from build123d import *

# Parameters (mm, degrees)
PAD_START          = -51
SKETCH_R           = 20
SKETCH_R_2         = 18.4
PAD_DEPTH          = 18
SKETCH001_R        = 21
PAD001_DEPTH       = 1
SKETCH002_R        = 4
PAD002_DEPTH       = 8.8
POCKET_DEPTH       = 9.801
PAD003_DEPTH       = 0.5
PAD003_DEPTH_BACK  = 0.5
POLARPATTERN_COUNT = 6


with BuildPart() as part:
    # Sketch → Pad (new body)
    with BuildSketch(Plane.XZ.offset(PAD_START)):
        Circle(SKETCH_R)
        Circle(SKETCH_R_2, mode=Mode.SUBTRACT)
    extrude(amount=-PAD_DEPTH)

    # Sketch001 (on Face3 of Pad) → Pad001 (join)
    with BuildSketch(Plane(origin=(0, 69, 0), x_dir=(1, 0, 0), z_dir=(0, 1, 0))):
        Circle(SKETCH001_R)
    extrude(amount=PAD001_DEPTH)

    # Sketch002 (on Face7 of Pad001) → Pad002 (join)
    with BuildSketch(Plane.XZ.offset(-69)):
        Circle(SKETCH002_R)
    extrude(amount=PAD002_DEPTH)

    # Sketch003 (on Face9 of Pad002) → Pocket (cut, through all)
    with BuildSketch(Plane.XZ.offset(-60.2)):
        with BuildLine():
            ThreePointArc((-1.249, 1), (-1.548005, -0.404574), (-0.6, -1.48324))
            Line((-0.6, -1.48324), (-0.6, -13.48324))
            Line((-0.6, -13.48324), (0.6, -13.48324))
            Line((0.6, -13.48324), (0.6, -1.48324))
            ThreePointArc((0.6, -1.48324), (1.548005, -0.404574), (1.249, 1))
            Line((-1.249, 1), (1.249, 1))
        make_face()
    extrude(amount=-POCKET_DEPTH, mode=Mode.SUBTRACT)

    # Sketch004 → Pad003 (join, two sides)
    with BuildSketch(Plane.XY) as pad003_sk:
        with BuildLine():
            ThreePointArc((-4, 60.2), (-5.757359, 64.442641), (-10, 66.2))
            ThreePointArc((-12.196813, 66.402796), (-11.103077, 66.250807), (-10, 66.2))
            Line((-19.7, 67.8), (-12.196813, 66.402796))
            Line((-19.7, 69), (-19.7, 67.8))
            Line((-19.7, 69), (-3.5, 69))
            Line((-3.5, 69), (-3.5, 60.2))
            Line((-3.5, 60.2), (-4, 60.2))
        make_face()
    pad003 = extrude(amount=PAD003_DEPTH) + extrude(pad003_sk.sketch, amount=-PAD003_DEPTH_BACK)

    # PolarPattern: Pad003 ×6 about axis
    polarpattern_axis = Axis((0, 0, 0), (0, 1, 0))
    for i in range(1, POLARPATTERN_COUNT):
        add(pad003.rotate(polarpattern_axis, i * 360 / POLARPATTERN_COUNT))


solid = part.part
The model under review builds one solid part; all positions refer to its coordinate system, in mm. A direction names the side the tool comes from. Give positions to 0.01 mm unless a question says otherwise; leave off trailing zeros. Write each loop counter-clockwise with the first axis right and the second up, starting at its lowest first coordinate (ties: lowest second). Pieces come first, ordered by that corner, then holes.
1. Add section A-A, the plane z = 0. Write out the cut boundary in (x, y).
2. Add section C-C, the plane y = 60.75. Count the separate pieces of the cut face and the enclosed holes in it, plus the area to 3 significant figures.
3. Wall thickness on L1, parallel to Z at x = 0, y = 60.5; L2, parallel to Z at x = 1, y = 66.5; L3, parallel to Z at x = 0, y = 58.5: over which ranges is each line inside the solid? List them lowest first.
4. Add section B-B, the plane x = 0. Write out the cut boundary in (y, z), plus the area to 3 significant figures.
5. Tool access review of faces 1 (the flat face through (-0.2, 60.2, 1.2)), 2 (the flat face through (18, 51, -6)), 3 (the flat face through (0, 69.5, -13.483)): name each direction out of +Z, -Z, +X, -X, +Y, -Y from which nothing blocks a thin tool from reaching the whole face with its end or side.
6. For P1, Ø5, axis at x = 7.5, y = 57.5, coming from the -Z side; P2, Ø2.5, axis at x = 13.5, y = 64, coming from the -Z side; P3, Ø4.5, axis at x = 3, z = 9.5, coming from the -Y side, all flat-tipped, find the tip position at first contact; note any pin that passes through.
7. Draft analysis for pull direction X (two halves, no side actions). For faces 4 (the cylindrical face through (-4.336, 59.874, -19.524)), 5 (the flat face through (-5.21, 67.23, 8.02)), 6 (the flat face through (0, 70, 4)), state which applies: +X half, -X half, draft (parallel to the pull), parting line (faces both ways), or undercut.
Worked answers:
1. outline: (-21, 69) - (-20, 69) - (-20, 51) - (-18.4, 51) - (-18.4, 67.56) - (-12.2, 66.4) arc R12 ccw to (-10, 66.2) arc R6 cw to (-4, 60.2) - (-1.6, 60.2) - (-1.6, 70) - (-21, 70) - close; (1.6, 60.2) - (4, 60.2) arc R6 cw to (10, 66.2) arc R12 ccw to (12.2, 66.4) - (18.4, 67.56) - (18.4, 51) - (20, 51) - (20, 69) - (21, 69) - (21, 70) - (1.6, 70) - close
2. separate pieces: 2
2. enclosed holes: 1
2. area: 234 mm2
3. L1: z = -20 to -18.4, 1 to 4, 18.4 to 20
3. L2: z = -19.97 to -18.37, -3.87 to -1.25, 1 to 3.87, 18.37 to 19.97
3. L3: z = -20 to -18.4, 18.4 to 20
4. outline: (51, -20) - (69, -20) - (69, -21) - (70, -21) - (70, -13.48) - (69, -13.48) - (69, -18.4) - (51, -18.4) - close; (51, 18.4) - (69, 18.4) - (69, 4) - (60.2, 4) - (60.2, 1) - (70, 1) - (70, 21) - (69, 21) - (69, 20) - (51, 20) - close
4. area: 112 mm2
5. face 1: -Y
5. face 2: +Z, -Z, +X, -X, -Y
5. face 3: +Y, -Y
6. P1: stops at z = -19.36
6. P2: stops at z = -15.81
6. P3: stops at y = 65.92
7. face 4: parting line
7. face 5: undercut
7. face 6: draft
